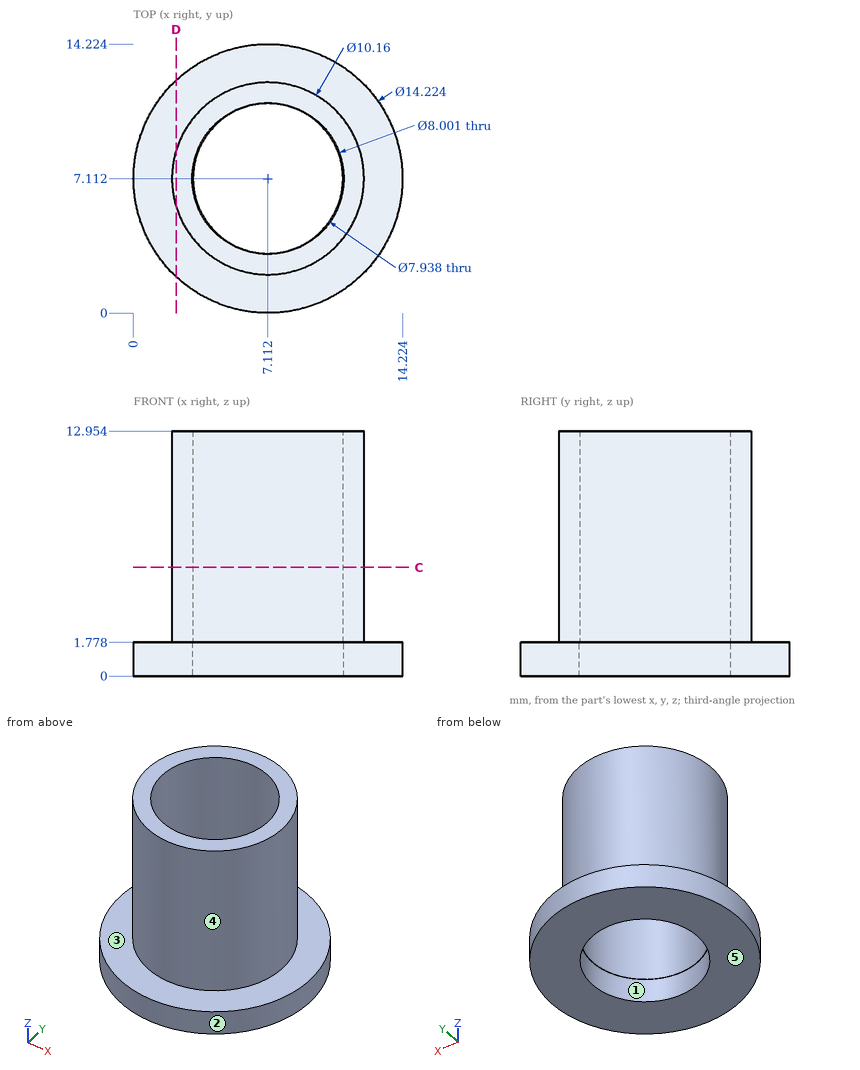
Here's the drawing with two shaded views (mm, measured from the low corner). I have some questions. A direction names the side the tool comes from. Round coordinates to 2 decimals unless told otherwise and drop trailing zeros. Write each loop counter-clockwise with the first axis right and the second up, starting at its lowest first coordinate (ties: lowest second). Pieces come first, ordered by that corner, then holes.
(1) Suppose I cut it at C-C on z = 5.75. Write out the boundary of the cut face in (x, y).
Findings below:
outline: circle Ø10.16 at (7.11, 7.11); hole circle Ø7.94 at (7.11, 7.11)
(2) Suppose I cut it at D-D on x = 2.25. Write out the boundary of the cut face in (y, z) (1 decimal).
Findings below:
outline: (1.9, 0) - (12.3, 0) - (12.3, 1.8) - (8.6, 1.8) - (8.6, 13) - (5.6, 13) - (5.6, 1.8) - (1.9, 1.8) - close
(3) Thinking about a two-plate mould opening in X: for the marked faces 1, 2 and 3, which applies, +X half, -X half, draft (parallel to the pull), parting line (faces both ways), or undercut?
Findings below:
face 1: undercut
face 2: parting line
face 3: draft
(4) For pin 1 (4 mm diameter, centred on y = 6, z = 8, fed in from -X); pin 2 (6.5 mm diameter, centred on x = 7, y = 7.5, fed in from -Z) (3 decimals); pin 3 (6 mm diameter, centred on x = 2, z = 1.5, fed in from +Y); pin 4 (5 mm diameter, centred on x = 3.5, z = 8.5, fed in from +Y), each with a flat end and sliding along its axis, tell me the tip position at first contact or that it passes through.
Findings below:
pin 1: stops at x = 2.03
pin 2: passes through
pin 3: stops at y = 13.9
pin 4: stops at y = 12.07
(5) If I drill on probe 1 along Z at (x, y) = (6.5, 0.75); probe 2 along Y at (x, z) = (9, 6) (1 decimal); probe 3 along Y at (x, z) = (3.5, 7) (1 decimal), over which ranges is the centre line in solid material (lowest first)?
Findings below:
probe 1: z = 0 to 1.78
probe 2: y = 2.4 to 3.6, 10.6 to 11.8
probe 3: y = 3.5 to 5.5, 8.8 to 10.7
(6) Which directions (+Z, -Z, +X, -X, +Y, -Y) give clear straight access to the entire face, cutting with the end or side of a thin tool? Please do the marked faces 4 and 5.
Findings below:
face 4: +Z
face 5: -Z, +X, -X, +Y, -Y
